from build123d import *

# Parameters (mm, degrees)
SKETCH1_W                    = 45.3
SKETCH1_H                    = 45.3
SKETCH1_W_2                  = 25
SKETCH1_H_2                  = 25
BOSS_EXTRUDE1_DEPTH          = 3
BOSS_EXTRUDE2_DEPTH          = 10.3
BOSS_EXTRUDE3_DEPTH          = 2.5
CIRPATTERN1_COUNT            = 3
CIRPATTERN1_ANGLE            = 180
CUT_EXTRUDE1_DEPTH           = 5
CUT_EXTRUDE1_DRAFT           = -10
CUT_EXTRUDE1_PROFILE_2_DEPTH = 5
CUT_EXTRUDE1_PROFILE_2_DRAFT = -10
CUT_EXTRUDE2_REACH           = 45.173


with BuildPart() as part:
    # Sketch1 → Boss-Extrude1 (new body)
    # profile 1 of 2: a face of its own
    with BuildSketch(Plane(origin=(0, 0, 0), x_dir=(1, 0, 0), z_dir=(0, 1, 0))):
        Polygon((-27.65, 22.65), (-22.65, 22.65), (-22.65, -22.65), (22.65, -22.65), (22.65, 22.65), (27.65, 22.65), (27.65, -27.65), (-27.65, -27.65), align=None)
    # profile 2 of 2: a face of its own
    with BuildSketch(Plane(origin=(0, 0, 0), x_dir=(1, 0, 0), z_dir=(0, 1, 0))):
        Rectangle(SKETCH1_W, SKETCH1_H)
        Rectangle(SKETCH1_W_2, SKETCH1_H_2, mode=Mode.SUBTRACT)
    extrude(amount=BOSS_EXTRUDE1_DEPTH)

    # Sketch1<3> → Boss-Extrude2 (add)
    with BuildSketch(Plane(origin=(0, 0, 0), x_dir=(1, 0, 0), z_dir=(0, 1, 0))):
        Polygon((-27.65, 22.65), (-22.65, 22.65), (-22.65, -22.65), (22.65, -22.65), (22.65, 22.65), (27.65, 22.65), (27.65, -27.65), (-27.65, -27.65), align=None)
    extrude(amount=-BOSS_EXTRUDE2_DEPTH)

    # Sketch2 → Boss-Extrude3 (add, symmetric)
    with BuildSketch(Plane(origin=(0, 0, 0), x_dir=(-1, 0, 0), z_dir=(0, 0, -1))):
        Polygon((-21.65, -12.3), (-24.65, -15.3), (-27.65, -15.3), (-27.65, -10.3), (-22.65, -10.3), (-21.65, -11.3), align=None)
    boss_extrude3 = extrude(amount=BOSS_EXTRUDE3_DEPTH, both=True)

    # CirPattern1: Boss-Extrude3 ×3 about axis
    cirpattern1_axis = Axis((0, 0, 0), (0, -1, 0))
    for i in range(1, CIRPATTERN1_COUNT):
        add(boss_extrude3.rotate(cirpattern1_axis, i * CIRPATTERN1_ANGLE / (CIRPATTERN1_COUNT - 1)))


with BuildPart() as cut_extrude1_tool:
    # Sketch3 → Cut-Extrude1 (with draft: the straight prism first)
    with BuildSketch(Plane.XZ.offset(10.3)):
        Polygon((21.65, 21.65), (21.65, 19.569375153), (28.65, 25.169375153), (28.65, 28.65), (25.169375153, 28.65), (19.569375153, 21.65), align=None)
    extrude(amount=-CUT_EXTRUDE1_DEPTH)
    # Cut-Extrude1: the draft: its side faces are tilted about the plane it starts from
    cut_extrude1_sides = [cut_extrude1_tool.faces().sort_by_distance(p)[0] for p in [
        (21.65, -7.8, 20.609687576),
        (25.15, -7.8, 22.369375153),
        (28.65, -7.8, 26.909687576),
        (26.909687576, -7.8, 28.65),
        (22.369375153, -7.8, 25.15),
        (20.609687576, -7.8, 21.65),
    ]]
    draft(cut_extrude1_sides, Plane.XZ.offset(10.3), CUT_EXTRUDE1_DRAFT)


with BuildPart() as part_1:
    add(part.part)

    # Cut-Extrude1: cut by cut_extrude1_tool
    add(cut_extrude1_tool.part, mode=Mode.SUBTRACT)


with BuildPart() as cut_extrude1_profile_2_tool:
    # Sketch3 → Cut-Extrude1 profile 2 (with draft: the straight prism first)
    with BuildSketch(Plane.XZ.offset(10.3)):
        Polygon((-21.65, 19.569375153), (-21.65, 21.65), (-19.569375153, 21.65), (-25.169375153, 28.65), (-28.65, 28.65), (-28.65, 25.169375153), align=None)
    extrude(amount=-CUT_EXTRUDE1_PROFILE_2_DEPTH)
    # Cut-Extrude1 profile 2: the draft: its side faces are tilted about the plane it starts from
    cut_extrude1_profile_2_sides = [cut_extrude1_profile_2_tool.faces().sort_by_distance(p)[0] for p in [
        (-21.65, -7.8, 20.609687576),
        (-20.609687576, -7.8, 21.65),
        (-22.369375153, -7.8, 25.15),
        (-26.909687576, -7.8, 28.65),
        (-28.65, -7.8, 26.909687576),
        (-25.15, -7.8, 22.369375153),
    ]]
    draft(cut_extrude1_profile_2_sides, Plane.XZ.offset(10.3), CUT_EXTRUDE1_PROFILE_2_DRAFT)


with BuildPart() as part_2:
    add(part_1.part)

    # Cut-Extrude1 profile 2: cut by cut_extrude1_profile_2_tool
    add(cut_extrude1_profile_2_tool.part, mode=Mode.SUBTRACT)

    # Sketch5 → Cut-Extrude2 (cut, up to next)
    with BuildSketch(Plane(origin=(0, 3, 0), x_dir=(1, 0, 0), z_dir=(0, 1, 0)), mode=Mode.PRIVATE) as cut_extrude2_sk1:
        with BuildLine():
            Line((15, 22.65), (-15, 22.65))
            ThreePointArc((-15, 22.65), (0, 19.65), (15, 22.65))
        make_face()
    cut_extrude2_tool1 = extrude(cut_extrude2_sk1.sketch, amount=-CUT_EXTRUDE2_REACH, mode=Mode.PRIVATE) & part_2.part
    add(cut_extrude2_tool1.solids().sort_by_distance((0, 3, -21.445954))[0], mode=Mode.SUBTRACT)


solid = part_2.part
Check sheet for the modelled part. Datum: model origin and axes. Units: mm. A direction names the side the tool comes from. Give positions to 0.01 mm unless a question says otherwise; leave off trailing zeros. Order: outer loops, then holes, each group sorted by start corner. A loop starts at its lowest first (then second) coordinate and runs counter-clockwise, first axis right, second up. Notation, with made-up numbers: (12.5, 6.5) - (21.5, 6.5) arc R19 ccw to (21.5, 22.5) - close; hole circle Ø1 at (-14.5, -28). An arc over 180 degrees is marked (long way). Answer as CSV lines item,"result".
1. Tool access check on faces 1 (the face through (25, -13, 2.5)), 2 (the face through (-25.193, -7.835, 22.96)), 3 (the face through (-23.13, -13.78, 0.04)), 4 (the face through (25, -10.3, -13)). Record the directions out of +Z, -Z, +X, -X, +Y, -Y that give a thin tool (end or side, any length) a straight path to the whole face; none if there is none.
Result sheet:
face 1,"+Z, +X, -X, -Y"
face 2,"-Y"
face 3,"+Z, -Z, -Y"
face 4,"-Z, +X, -X, -Y"
2. Go/stop test with flat-tipped pins: P1, Ø10, axis at x = -5.5, z = -4, coming from the +Y side; P2, Ø4, axis at x = -24.5, y = -12.5, coming from the -Z side; P3, Ø2.5, axis at x = -25, z = -8, coming from the -Y side; P4, Ø0.8, axis at x = 0, y = -11.5, coming from the -Z side. Record where each tip stops, or that it passes through.
Result sheet:
P1,"through"
P2,"z = -2.5"
P3,"y = -10.3"
P4,"z = 21.65"
3. Section check C-C (x = -4). Record the boundary of the cut face in (y, z).
Result sheet:
outline,"(-10.3, 22.65) - (0, 22.65) - (0, 12.5) - (3, 12.5) - (3, 27.65) - (-10.3, 27.65) - close; (0, -19.86) - (3, -19.86) - (3, -12.5) - (0, -12.5) - close"
4. Scan lines: probe 1 along X at (y, z) = (0.5, 8.5); probe 2 along X at (y, z) = (-7.5, -11.5); probe 3 along Y at (x, z) = (-24.5, 5). Record each from-to range of solid material in increasing order. Write a range as from..to.
Result sheet:
probe 1,"-27.65..-12.5, 12.5..27.65"
probe 2,"-27.65..-22.65, 22.65..27.65"
probe 3,"-10.3..3"
5. Section check B-B (y = -7.5). Record the boundary of the cut face in (x, z), then the cut area to 3 significant figures.
Result sheet:
outline,"(-27.65, -22.65) - (-22.65, -22.65) - (-22.65, 21) - (-27.65, 25) - close; (-25, 27.65) - (-21, 22.65) - (21, 22.65) - (25, 27.65) - close; (22.65, -22.65) - (27.65, -22.65) - (27.65, 25) - (22.65, 21) - close"
area,"687 mm²"
6. Section check A-A (z = -8). Record the boundary of the cut face in (x, y), then the cut area to 3 significant figures.
Result sheet:
outline,"(-27.65, -10.3) - (-22.65, -10.3) - (-22.65, 0) - (-12.5, 0) - (-12.5, 3) - (-27.65, 3) - close; (12.5, 0) - (22.65, 0) - (22.65, -10.3) - (27.65, -10.3) - (27.65, 3) - (12.5, 3) - close"
area,"194 mm²"
7. Section check D-D (z = -16.5). Record the boundary of the cut face in (x, y).
Result sheet:
outline,"(-27.65, -10.3) - (-22.65, -10.3) - (-22.65, 0) - (22.65, 0) - (22.65, -10.3) - (27.65, -10.3) - (27.65, 3) - (-27.65, 3) - close"
8. Mould release check, pull along X, two halves, no side actions. Record for faces 5 (the face through (22.65, -5, 0)), 6 (the face through (25, -10.3, 13)), 7 (the face through (27.65, -4, 2)): released by +X, released by -X, zero draft, split by the parting line, or undercut.
Result sheet:
face 5,"undercut"
face 6,"zero draft"
face 7,"released by +X"
